Autodesk Inventor part; units mm, degrees
ref_plane "YZ Plane" through (0, 0, 0) normal (1, 0, 0) x (0, 1, 0)
ref_plane "XZ Plane" through (0, 0, 0) normal (0, 1, 0) x (-1, 0, 0)
ref_plane "XY Plane" through (0, 0, 0) normal (0, 0, 1) x (1, 0, 0)
sketch "Sketch1" plane through (0, 0, 0) normal (0, 0, 1) x (1, 0, 0)
  circle A0 centre (0, 0) radius 4.51
  circle A1 centre (0, 0) radius 8.4
  dimension "d0" = 9.02
  dimension "d1" = 16.8
extrude "Extrusion1" add sketch "Sketch1" along normal blind 5
sketch "Sketch2" plane through (0, 0, 5) normal (0, 0, 1) x (1, 0, 0)
  line L0 (-7.5, 7.5) -> (7.5, 7.5)
  line L1 (7.5, 7.5) -> (7.5, -7.5)
  line L2 (7.5, -7.5) -> (-7.5, -7.5)
  line L3 (-7.5, -7.5) -> (-7.5, 7.5)
  line L4 (0, 0) -> (0, 8.3867)
  line L5 (0, 0) -> (9.7878, 0)
  circle A0 centre (0, 0) radius 10.6066
  point P0 (0, 7.5)
  point P1 (7.5, 0)
  dimension "d4" = 15
extrude "Extrusion2" cut sketch "Sketch2" against normal blind 3 contours A0 L0 | L3 A0 | L2 A0 | A0 L1
properties part number "TuercaD_eje" material "Steel"
The model under review builds one solid part; all positions refer to its coordinate system, in mm. A direction names the side the tool comes from. Round coordinates to 2 decimals unless told otherwise and drop trailing zeros. Write each loop counter-clockwise with the first axis right and the second up, starting at its lowest first coordinate (ties: lowest second). Pieces come first, ordered by that corner, then holes. Notation, with made-up numbers: M 86,-10.75 L 140,-10.75 A20 ccw 140,27.25 Z; hole C -10,61.25 d9. An arc over 180 degrees is marked long. Use CSV: the item, a comma, the result in double quotes. Start each with the question number.
(1) For line 1 along Y through (x, z) = (0, 1.5); line 2 along Y through (x, z) = (0, 3.55); line 3 along X through (y, z) = (-3, 3.8), list the stretches that pass through material, from the lowest coordinate up.
(2) We need section D-D, the plane z = 0.7. State the section outline as (x, y) points.
(3) Clearance check with flat-ended pins moving along their axes: P1, Ø1.5, axis at y = 4.5, z = 3, coming from the +X side; P2, Ø2, axis at x = -5.5, z = 2, coming from the -Y side; P3, Ø0.7, axis at x = -0.5, y = -8, coming from the +Z side; P4, Ø8, axis at x = 0, y = 0, coming from the -Z side. State where each tip first meets the part, or that it passes through.
(4) The part is to be moulded in two halves that separate along Y. For faces 5 (the face through (0, -8, 2)), 6 (the face through (0, 7.5, 4)), 7 (the face through (-8.39, -0.37, 1.35)), 8 (the face through (4.166, 1.727, 2.465)), say which applies: +Y half, -Y half, draft (parallel to the pull), parting line (faces both ways), or undercut.
(5) We need section A-A, the plane y = 0. State the section outline as (x, z) points, then the cut area to 3 significant figures.
(6) Tool access review of faces 1 (the face through (0, -7.5, 4)), 2 (the face through (0, 8, 2)), 3 (the face through (7.5, 0, 4)), 4 (the face through (-7.5, 0, 4)): name each direction out of +Z, -Z, +X, -X, +Y, -Y from which nothing blocks a thin tool from reaching the whole face with its end or side.
(7) We need section C-C, the plane z = 4.2. State the section outline as (x, y) points, then the cut area to 3 significant figures.
Findings:
1,line 1,"-8.4 to -4.51, 4.51 to 8.4"
1,line 2,"-7.5 to -4.51, 4.51 to 7.5"
1,line 3,"-7.5 to -3.37, 3.37 to 7.5"
2,outline,"C 0,0 d16.8; hole C 0,0 d9.02"
3,P1,"x = 7.5"
3,P2,"y = -7.09"
3,P3,"z = 2"
3,P4,"through"
4,face 5,"draft"
4,face 6,"+Y half"
4,face 7,"parting line"
4,face 8,"undercut"
5,outline,"M -8.4,0 L -4.51,0 L -4.51,5 L -7.5,5 L -7.5,2 L -8.4,2 Z; M 4.51,0 L 8.4,0 L 8.4,2 L 7.5,2 L 7.5,5 L 4.51,5 Z"
5,area,"33.5 mm^2"
6,face 1,"+Z, +X, -X, -Y"
6,face 2,"+Z, +X, -X, +Y"
6,face 3,"+Z, +X, +Y, -Y"
6,face 4,"+Z, -X, +Y, -Y"
7,outline,"M -7.5,-3.78 A8.4 ccw -3.78,-7.5 L 3.78,-7.5 A8.4 ccw 7.5,-3.78 L 7.5,3.78 A8.4 ccw 3.78,7.5 L -3.78,7.5 A8.4 ccw -7.5,3.78 Z; hole C 0,0 d9.02"
7,area,"139 mm^2"
